Autodesk Inventor part; units mm, degrees
ref_plane "YZ Plane" through (0, 0, 0) normal (1, 0, 0) x (0, 1, 0)
ref_plane "XZ Plane" through (0, 0, 0) normal (0, 1, 0) x (-1, 0, 0)
ref_plane "XY Plane" through (0, 0, 0) normal (0, 0, 1) x (1, 0, 0)
sketch "Sketch12" plane through (0, 0, 0) normal (0, 0, 1) x (1, 0, 0)
  line L0 (0, 0) -> (35, 0)
  line L1 (35, 0) -> (35, 47)
  line L2 (35, 47) -> (0, 47)
  line L3 (0, 47) -> (0, 0)
  line L4 (0, 47) -> (2, 47) construction
  line L5 (2, 47) -> (2, 35.5) construction
  line L6 (35, 47) -> (33, 47) construction
  line L7 (33, 47) -> (33, 35.5) construction
  circle A0 centre (33, 35.5) radius 1.25
  circle A1 centre (2, 35.5) radius 1.25
  line L8 (0, 0) -> (6.5, 0) construction
  line L9 (35, 0) -> (28.5, 0) construction
  line L10 (6.5, 0) -> (6.5, 3.2) construction
  line L11 (28.5, 0) -> (28.5, 3.2) construction
  circle A2 centre (28.5, 3.2) radius 1.25
  dimension "d49" = 35
  dimension "d50" = 47
  dimension "d97" = 2
  dimension "d98" = 11.5
  dimension "d99" = 2
  dimension "d100" = 2.5
  dimension "d101" = 2.5
  dimension "d102" = 11.5
  dimension "d103" = 6.5
  dimension "d104" = 6.5
  dimension "d105" = 3.2
  dimension "d106" = 3.2
  dimension "d108" = 2.5
extrude "Extrusión8" add sketch "Sketch12" along normal blind 1
sketch "Sketch25" plane through (0, 47, 0) normal (0, 1, 0) x (1, 0, 0)
  point P0 (0, 0)
sketch "Sketch26" plane through (0, 0, 0) normal (0, -1, 0) x (1, 0, 0)
  line L0 (35, 1) -> (20.1754, 1)
  line L1 (20.1754, 1) -> (20.1754, 15)
  line L2 (20.1754, 15) -> (35, 15)
  line L3 (35, 15) -> (35, 1)
  line L4 (0, 1) -> (14.825, 1)
  line L5 (35, 1) -> (0, 1)
  line L6 (14.825, 1) -> (14.825, 15)
  line L7 (14.825, 15) -> (0, 15)
  line L8 (0, 15) -> (0, 1)
  point P0 (0, 0)
  dimension "d121" = 14.825
  dimension "d126" = 14
extrude "Extrusion10" add sketch "Sketch26" against normal blind 1 contours L4 L8 L7 L6
fillet "Empalme1" radius 2 1 edges at (7.4125, 1, 1)
sketch "Boceto28" plane through (0, 47, 0) normal (0, 1, 0) x (1, 0, 0)
  line L0 (0, 0) -> (0, -1)
  line L1 (0, -1) -> (14.825, -1)
  line L2 (0, -3) -> (14.825, -3)
  line L3 (14.825, -15) -> (14.825, -3)
  line L4 (14.825, -1) -> (14.825, -15)
  line L5 (0, -15) -> (14.825, -15)
  line L6 (14.825, -15) -> (0, -15)
  line L7 (0, -15) -> (0, -1)
  point P0 (14.825, -3)
extrude "Extrusión12" add sketch "Boceto28" against normal blind 1
fillet "Empalme2" radius 2 1 edges at (7.4125, 46, 1)
sketch "Boceto29" plane through (0, 47, 0) normal (0, 1, 0) x (1, 0, 0)
  line L0 (0, 0) -> (0, -15)
  line L1 (0, -7.5) -> (14.825, -7.5)
  line L2 (14.825, -15) -> (14.825, -3)
  line L3 (7.4125, -7.5) -> (7.4125, -15)
  line L4 (0, -15) -> (14.825, -15)
  circle A0 centre (7.4125, -7.5) radius 1.5
  dimension "d127" = 3
extrude "Extrusión13" cut sketch "Boceto29" against normal through all contours A0 L1 | L1 L3 A0 | L1 A0 L3
equation "\"BendRadius\" = Thickness"
equation "\"BendReliefWidth\" = Thickness"
equation "\"BendReliefDepth\" = 0.5 * Thickness"
equation "\"CornerReliefSize\" = 4 * Thickness"
equation "\"MinimumRemnant\" = 2 * Thickness"
equation "\"TransitionRadius\" = BendRadius"
equation "\"JacobiRadiusSize\" = BendRadius"
equation "\"GapSize\" = Thickness"
properties part number "Suportmotor"
CAD build for the part. Positions are in the model's coordinates, mm. A direction names the side the tool comes from. Give positions to 0.01 mm unless a question says otherwise; leave off trailing zeros. Order: outer loops, then holes, each group sorted by start corner. A loop starts at its lowest first (then second) coordinate and runs counter-clockwise, first axis right, second up.
(1) Saw through at D-D, the plane z = 3.5. Give the cut face in (x, y) (3 decimals), then the cut area to 4 significant figures.
(2) Saw through at A-A, the plane z = 7.5. Give the cut face in (x, y) (1 decimal), then the cut area to 4 significant figures.
(3) Saw through at C-C, the plane y = 35.5. Give the cut face in (x, z), then the cut area to 3 significant figures.
(4) Saw through at B-B, the plane x = 28.5. Give the cut face in (y, z), then the cut area to 3 significant figures.
(5) Tool access for faces 4 (the flat face through (7, 46, 10)), 5 (the flat face through (17, 24, 0)), 6 (the flat face through (14.825, 0.5, 7.4)): list every direction of +Z, -Z, +X, -X, +Y, -Y with a clear straight run to the whole face (end or side of a thin tool).
(6) Flat gauge pins, fed straight in: pin 1 (8 mm diameter, centred on x = 7, y = 6, fed in from +Z); pin 2 (3 mm diameter, centred on x = 4.5, y = 34, fed in from -Z); pin 3 (2.5 mm diameter, centred on y = 45, z = 11.5, fed in from +X) (3 decimals); pin 4 (12 mm diameter, centred on x = 23.5, y = 17, fed in from +Z). Where does each tip first touch, or does it go through?
(7) Drill centre lines: L1, parallel to Y at x = 6, z = 3.5; L2, parallel to Y at x = 2, z = 0.45; L3, parallel to Z at x = 26.5, y = 23.5. Where is each one in solid material? Low to high.
(8) Mould opens along Y. For faces 1 (the flat face through (9, 0, 7)), 2 (the flat face through (35, 23.2, 0.5)), 3 (the cylindrical face through (33.577, 36.609, 0.493)) say: released by +Y, released by -Y, zero draft, split by the parting line, or undercut.
Results found:
1. outline: (0, 0) - (14.825, 0) - (14.825, 1) - (0, 1) - close; (0, 46) - (14.825, 46) - (14.825, 47) - (0, 47) - close
1. area: 29.65 mm2
2. outline: (0, 0) - (5.9, 0) - (5.9, 1) - (0, 1) - close; (0, 46) - (5.9, 46) - (5.9, 47) - (0, 47) - close; (8.9, 0) - (14.8, 0) - (14.8, 1) - (8.9, 1) - close; (8.9, 46) - (14.8, 46) - (14.8, 47) - (8.9, 47) - close
2. area: 23.65 mm2
3. outline: (0, 0) - (0.75, 0) - (0.75, 1) - (0, 1) - close; (3.25, 0) - (31.75, 0) - (31.75, 1) - (3.25, 1) - close; (34.25, 0) - (35, 0) - (35, 1) - (34.25, 1) - close
3. area: 30.0 mm2
4. outline: (0, 0) - (1.95, 0) - (1.95, 1) - (0, 1) - close; (4.45, 0) - (47, 0) - (47, 1) - (4.45, 1) - close
4. area: 44.5 mm2
5. face 4: +Z, +X, -X
5. face 5: -Z, +X, -X, +Y, -Y
5. face 6: +Z, +X, +Y, -Y
6. pin 1: stops at z = 1.27
6. pin 2: stops at z = 0
6. pin 3: stops at x = 14.825
6. pin 4: stops at z = 1
7. L1: y = 0 to 1, 46 to 47
7. L2: y = 0 to 34.25, 36.75 to 47
7. L3: z = 0 to 1
8. face 1: released by -Y
8. face 2: zero draft
8. face 3: undercut
